Verification items for the finished model (mm, model axes). Round coordinates to 2 decimals unless told otherwise and drop trailing zeros. Write each loop counter-clockwise with the first axis right and the second up, starting at its lowest first coordinate (ties: lowest second). Pieces come first, ordered by that corner, then holes. Notation, with made-up numbers: M 73,51.5 L 99,51.5 A20 cw 99,60.5 Z; hole C -28.75,51.25 d11. An arc over 180 degrees is marked long. One line per item, written item: value. Start each with the question number.
Item 1: Section check C-C, the plane x = 223.5. Record the cut outline in (y, z), then the cut area to 3 significant figures.
Item 2: Thickness scan on probe 1 along Z at (x, y) = (-37.5, 2); probe 2 along Z at (x, y) = (-30, 0.3); probe 3 along X at (y, z) = (1.7, -140). Record the ranges inside material, lowest first. Write a range as from..to.
Item 3: Section check A-A, the plane y = 4.2. Record the cut outline in (x, z), then the cut area to 3 significant figures.
Item 4: Section check B-B, the plane z = 205. Record the cut outline in (x, y), then the cut area to 3 significant figures.
Item 5: Gauge pin test, flat end, axial feed: pin 1 (3 mm diameter, centred on x = -210, y = 3.5, fed in from +Z). Record the tip position at first contact, or that the pin passes through.
from build123d import *

# Parameters (mm, degrees)
ESBO_O1_R                  = 275
RESSALTO_EXTRUS_O1_DEPTH   = 6
FURO_DE_DI_METRO_6_0_6_1_D = 6


with BuildPart() as part:
    # Esboço1 → Ressalto-extrusão1 (new body)
    with BuildSketch(Plane(origin=(0, 0, 0), x_dir=(1, 0, 0), z_dir=(0, 1, 0))):
        with Locations(Location((0, 0, 0), (0, 0, 270))):
            Circle(ESBO_O1_R)
    extrude(amount=RESSALTO_EXTRUS_O1_DEPTH)

    # Furo de diâmetro Ø6.0 (6)1 (through all)
    with Locations(Plane(origin=(0, 6, 0), x_dir=(1, 0, 0), z_dir=(0, 1, 0))):
        with Locations((0, 37.5), (37.5, 0), (0, -37.5), (-37.5, 0)):
            Hole(FURO_DE_DI_METRO_6_0_6_1_D / 2)


solid = part.part
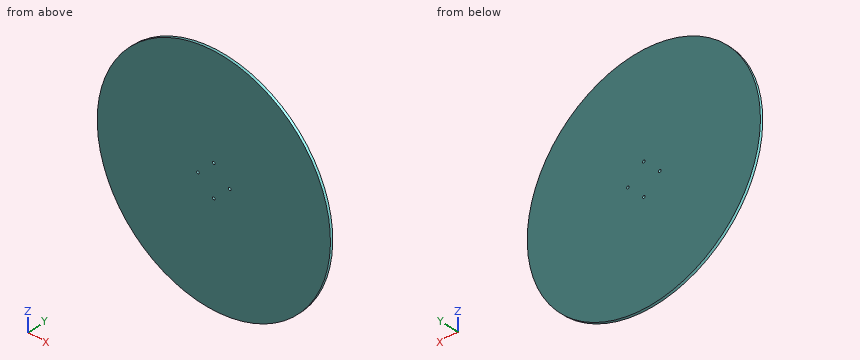
Response values:
1. outline: M 0,-160.23 L 6,-160.23 L 6,160.23 L 0,160.23 Z
1. area: 1,920 mm2
2. probe 1: z = -272.43..-3, 3..272.43
2. probe 2: z = -273.36..273.36
2. probe 3: x = -236.7..236.7
3. outline: C 0,0 d550; hole C -37.5,0 d6; hole C 0,-37.5 d6; hole C 0,37.5 d6; hole C 37.5,0 d6
3. area: 237,000 mm2
4. outline: M -183.3,0 L 183.3,0 L 183.3,6 L -183.3,6 Z
4. area: 2,200 mm2
5. pin 1: stops at z = 179.31
